Model file for the job. Use its own axes, mm. A direction names the side the tool comes from. Round coordinates to 2 decimals unless told otherwise and drop trailing zeros. Loops run counter-clockwise (first coordinate to the right, second up) from the corner with the lowest first, then second, coordinate; pieces in that order, holes last. Notation, with made-up numbers: (-35, -31) - (4, -31) arc R27 cw to (4, -1) - close; hole circle Ø3 at (47.5, 13.5). An arc over 180 degrees is marked (long way). Answer as a JSON object with one key per item and string values.
from build123d import *

# Parameters (mm, degrees)
SKETCH_R           = 42
SKETCH_R_2         = 20
PAD_DEPTH          = 10
SKETCH001_R        = 6
POCKET_DEPTH       = 10.001
POCKET001_DEPTH    = 248.429186
POLARPATTERN_COUNT = 8


with BuildPart() as part:
    # Sketch → Pad (new body)
    with BuildSketch(Plane.XY):
        Circle(SKETCH_R)
        Circle(SKETCH_R_2, mode=Mode.SUBTRACT)
    extrude(amount=PAD_DEPTH)

    # Sketch001 (on Face4 of Pad) → Pocket (cut, through all)
    with BuildSketch(Plane.XY.offset(10)):
        with Locations((-36.37, 21)):
            Circle(SKETCH001_R)
        with Locations((36.37, -21)):
            Circle(SKETCH001_R)
    extrude(amount=-POCKET_DEPTH, mode=Mode.SUBTRACT)

    # Sketch002 (on Face4 of Pocket) → Pocket001 (cut, through all)
    with BuildSketch(Plane.XY.offset(10)):
        with BuildLine():
            ThreePointArc((3, 24.803848), (0, 36), (-3, 24.803848))
            Line((-3, 24.803848), (-3, 19.77372))
            ThreePointArc((3, 19.77372), (0, 20), (-3, 19.77372))
            Line((3, 24.803848), (3, 19.77372))
        make_face()
    pocket001 = extrude(amount=-POCKET001_DEPTH, mode=Mode.SUBTRACT)

    # PolarPattern: Pocket001 ×8 about axis
    polarpattern_axis = Axis((0, 0, 10), (0, 0, 1))
    for i in range(1, POLARPATTERN_COUNT):
        add(pocket001.rotate(polarpattern_axis, i * 360 / POLARPATTERN_COUNT), mode=Mode.SUBTRACT)


solid = part.part
1) Two-plate mould, pull along X, no slides. Class faces 3 (the cylindrical face through (-21.72, -35.95, 4.93)), 4 (the flat face through (-10, -18, 10)), 5 (the flat face through (-17.907, -13.664, 5.07)): pulls with the +X half, pulls with the -X half, needs draft (parallel to the pull), parting line crosses it, or undercut.
Values follow:
{"face 3": "parting line crosses it", "face 4": "needs draft", "face 5": "undercut"}
2) Slice it at A-A on y = 0. List the corners of the cut face in (x, z), then the cut area to 3 significant figures.
Values follow:
{"outline": "(-42, 0) - (-36, 0) - (-36, 10) - (-42, 10) - close; (36, 0) - (42, 0) - (42, 10) - (36, 10) - close", "area": "120 mm²"}
3) Slice it at C-C on y = -21.5. List the corners of the cut face in (x, z), then the cut area to 3 significant figures.
Values follow:
{"outline": "(-36.08, 0) - (-27.21, 0) - (-27.21, 10) - (-36.08, 10) - close; (-15.22, 0) - (-3, 0) - (-3, 10) - (-15.22, 10) - close; (3, 0) - (15.22, 0) - (15.22, 10) - (3, 10) - close; (27.21, 0) - (30.39, 0) - (30.39, 10) - (27.21, 10) - close", "area": "365 mm²"}
4) Tool access for faces 1 (the flat face through (-10, -18, 0)), 2 (the flat face through (22, -3, 5)): list every direction of +Z, -Z, +X, -X, +Y, -Y with a clear straight run to the whole face (end or side of a thin tool).
Values follow:
{"face 1": "-Z, +X, -X, +Y, -Y", "face 2": "+Z, -Z"}
5) Slice it at B-B on x = -13.5. List the corners of the cut face in (y, z).
Values follow:
{"outline": "(-39.77, 0) - (-17.74, 0) - (-17.74, 10) - (-39.77, 10) - close; (17.74, 0) - (39.77, 0) - (39.77, 10) - (17.74, 10) - close"}
6) Probe probe 1 along X at (y, z) = (-21, 6.75); probe 2 along X at (y, z) = (16.5, 9.5); probe 3 along Y at (x, z) = (0, 4.75). List the from-to ranges inside material, lowest first.
Values follow:
{"probe 1": "-36.37 to -27.21, -15.22 to -3, 3 to 15.22, 27.21 to 30.37", "probe 2": "-32.4 to -24.93, -12.26 to -11.3, 11.3 to 12.26, 24.93 to 38.62", "probe 3": "-42 to -36, 36 to 42"}
7) Drop flat-ended pins along their axis: P1, Ø2.5, axis at x = 22, z = 3, coming from the -Y side; P2, Ø9.5, axis at x = -30, y = 0, coming from the -Z side; P3, Ø1.5, axis at y = -22.5, z = 2.5, coming from the -X side; P4, Ø1.5, axis at y = -24, z = 4.5, coming from the -X side. Give the stop position or say it passes through.
Values follow:
{"P1": "y = -36.52", "P2": "through", "P3": "x = -35.93", "P4": "x = -34.98"}
